Part model, mm, in its own coordinate system. Face numbers are marked on the shaded views. Round coordinates to 2 decimals unless told otherwise and drop trailing zeros. Write each loop counter-clockwise with the first axis right and the second up, starting at its lowest first coordinate (ties: lowest second). Pieces come first, ordered by that corner, then holes. Notation, with made-up numbers: M 12.5,27 L 62.5,27 A29 ccw 62.5,57 Z; hole C 58,-25.75 d1. An arc over 180 degrees is marked long. One line per question, with ' | ' between items. Start each with the question number.
1) Saw through at D-D (x = 18). List the corners of the cut face in (y, z), plus the area to 3 significant figures.
2) Saw through at C-C (z = -215.9). List the corners of the cut face in (x, y) (3 decimals), plus the area to 3 significant figures.
3) Mould opens along X. For the marked faces 1, 2 and 3 say: pulls with the +X half, pulls with the -X half, needs draft (parallel to the pull), parting line crosses it, or undercut.
4) Wall check: probe 1 along Z at (x, y) = (0, -6.25) (3 decimals); probe 2 along Y at (x, z) = (14, -63); probe 3 along X at (y, z) = (0, -127). Give the ranges that are in metal, low to high. Write a range as [from, to].
5) Saw through at B-B (y = 0). List the corners of the cut face in (x, z) (3 decimals).
6) Saw through at A-A (x = 0). List the corners of the cut face in (y, z) (3 decimals), plus the area to 3 significant figures.
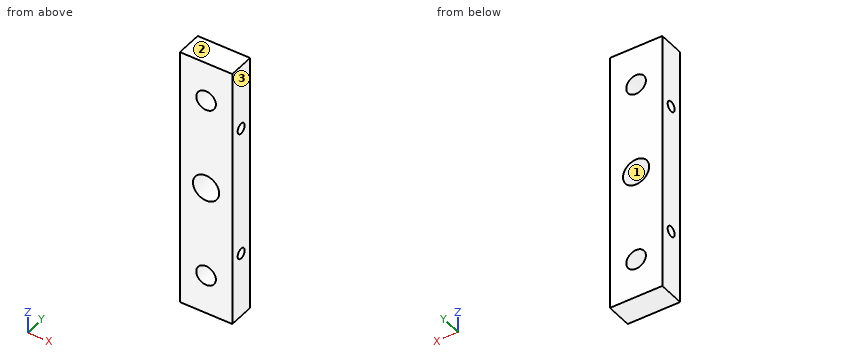
Autodesk Inventor part; units mm, degrees
ref_plane "YZ Plane" through (0, 0, 0) normal (1, 0, 0) x (0, 1, 0)
ref_plane "XZ Plane" through (0, 0, 0) normal (0, 1, 0) x (-1, 0, 0)
ref_plane "XY Plane" through (0, 0, 0) normal (0, 0, 1) x (1, 0, 0)
sketch "Sketch1" plane through (0, 0, 0) normal (0, 0, 1) x (1, 0, 0)
  line L0 (-25.4, -12.7) -> (25.4, -12.7)
  line L1 (25.4, -12.7) -> (25.4, 12.7)
  line L2 (25.4, 12.7) -> (-25.4, 12.7)
  line L3 (-25.4, 12.7) -> (-25.4, -12.7)
  line L4 (-25.4, -12.7) -> (25.4, 12.7) construction
  line L5 (25.4, -12.7) -> (-25.4, 12.7) construction
  point P0 (0, 0)
  dimension "d0" = 25.4
  dimension "d1" = 50.8
extrude "Extrusion1" add sketch "Sketch1" against normal blind 254
sketch "Sketch2" plane through (-25.4, 12.7, 0) normal (0, 1, 0) x (1, 0, 0)
  circle A0 centre (25.4, 38.1) radius 9.525
  circle A1 centre (25.4, 215.9) radius 9.525
  line L0 (50.8, 0) -> (0, 0)
  line L1 (0, 0) -> (0, 254)
  circle A2 centre (25.4, 127) radius 12.7
  point P0 (25.4, 0)
  point P1 (25.4, 0)
  point P2 (0, 127)
  point P3 (0, 127)
  dimension "d4" = 19.05
  dimension "d5" = 88.9
  dimension "d6" = 177.8
  dimension "d9" = 25.4
extrude "Extrusion2" cut sketch "Sketch2" against normal blind 254
sketch "Sketch3" plane through (25.4, -12.7, 0) normal (1, 0, 0) x (0, 0, -1)
  circle A0 centre (63.5, 12.7) radius 5
  circle A1 centre (190.5, 12.7) radius 5
  line L0 (0, 25.4) -> (254, 25.4)
  line L1 (0, 0) -> (0, 25.4)
  point P0 (0, 12.7)
  point P1 (127, 25.4)
  point P2 (0, 12.7)
  dimension "d10" = 10
  dimension "d11" = 127
  dimension "d12" = 63.5
extrude "Extrusion3" cut sketch "Sketch3" against normal blind 254
properties part number "Metal Bar-2"
Answer key:
1) outline: M -12.7,-254 L 12.7,-254 L 12.7,0 L -12.7,0 Z; hole C 0,-190.5 d10; hole C 0,-63.5 d10 | area: 6,290 mm2
2) outline: M -25.4,-12.7 L -9.525,-12.7 L -9.525,12.7 L -25.4,12.7 Z; M 9.525,-12.7 L 25.4,-12.7 L 25.4,12.7 L 9.525,12.7 Z | area: 806 mm2
3) face 1: undercut | face 2: needs draft | face 3: pulls with the +X half
4) probe 1: z = [-254, -225.425], [-206.375, -139.7], [-114.3, -47.625], [-28.575, 0] | probe 2: y = [-12.7, -4.97], [4.97, 12.7] | probe 3: x = [-25.4, -12.7], [12.7, 25.4]
5) outline: M -25.4,-254 L 25.4,-254 L 25.4,-195.5 L -25.4,-195.5 Z; M -25.4,-185.5 L 25.4,-185.5 L 25.4,-68.5 L -25.4,-68.5 Z; M -25.4,-58.5 L 25.4,-58.5 L 25.4,0 L -25.4,0 Z; hole C 0,-127 d25.4; hole C 0,-215.9 d19.05; hole C 0,-38.1 d19.05
6) outline: M -12.7,-254 L 12.7,-254 L 12.7,-225.425 L -12.7,-225.425 Z; M -12.7,-206.375 L 12.7,-206.375 L 12.7,-139.7 L -12.7,-139.7 Z; M -12.7,-114.3 L 12.7,-114.3 L 12.7,-47.625 L -12.7,-47.625 Z; M -12.7,-28.575 L 12.7,-28.575 L 12.7,0 L -12.7,0 Z; hole C 0,-190.5 d10; hole C 0,-63.5 d10 | area: 4,680 mm2
